from build123d import *

# Parameters (mm, degrees)
F0_W      = 50
F0_H      = 90
F1_DEPTH  = 50
F3_DEPTH  = 90.001
F4_R      = 8.198492098
F5_DEPTH  = 50.001
F6_R      = 10.8639610307
F8_DEPTH  = 50.001
F11_DEPTH = 90.001
F13_DEPTH = 90.0010001
F14_DEPTH = 90.0010001
F15_DEPTH = 27


with BuildPart() as f1:
    # F0 (on Top) → F1 (new body)
    with BuildSketch(Plane.XY):
        Rectangle(F0_W, F0_H)
    extrude(amount=F1_DEPTH)

    # F2 (on face) → F3 (cut, through all)
    with BuildSketch(Plane.XZ.offset(45)):
        Polygon((0, 25), (-25, 0), (25, 0), align=None)
    extrude(amount=-F3_DEPTH, mode=Mode.SUBTRACT)

    # F4 (on face) → F5 (cut, through all)
    with BuildSketch(Plane(origin=(-25, 0, 0), x_dir=(0, -1, 0), z_dir=(-1, 0, 0))):
        with Locations((-33.659145236, 38.9719307423)):
            Circle(F4_R)
    extrude(amount=-F5_DEPTH, mode=Mode.SUBTRACT)

    # F6
    f6_edges = [f1.edges().sort_by_distance(p)[0] for p in [
        (0, 45, 50),
    ]]
    fillet(f6_edges, radius=F6_R)

    # F7 (on face) → F8 (cut, through all)
    with BuildSketch(Plane.YZ.offset(25)):
        Polygon((28.1980223954, 0), (45, 0), (45, 29.2644444853), align=None)
    extrude(amount=-F8_DEPTH, mode=Mode.SUBTRACT)

    # F10 (on face) → F11 (cut, through all)
    with BuildSketch(Plane.XZ.offset(45)):
        with BuildLine():
            add(Edge.make_bspline(
                [(0, 46.1721457541), (-10.2533935373, 46.1721457541), (-5.1266967687, 31.8932551891), (0, 17.614364624), (5.1266967687, 31.8932551891), (10.2533935373, 46.1721457541), (0, 46.1721457541)],
                knots=[0, 0, 0, 2.0943951024, 2.0943951024, 4.1887902048, 4.1887902048, 6.2831853072, 6.2831853072, 6.2831853072], degree=2, weights=[1, 0.5, 1, 0.5, 1, 0.5, 1]))
        make_face()
    extrude(amount=-F11_DEPTH, mode=Mode.SUBTRACT)

    # F12 (on face) → F13 (cut, through all)
    with BuildSketch(Plane.XZ.offset(45)):
        Polygon((25, 7.2744810022), (17.7255189978, 7.2744810022), (25, 0), align=None)
        Polygon((-17.7255189978, 7.2744810022), (-25, 7.2744810022), (-25, 0), align=None)
    extrude(amount=-F13_DEPTH, mode=Mode.SUBTRACT)

    # F9 (on face) → F14 (cut, through all)
    with BuildSketch(Plane.XZ.offset(45)):
        Polygon((25, 10.9673021361), (25, 46.2542101741), (10.0381237455, 25.9291783907), align=None)
        Polygon((-25, 46.2542101741), (-25, 10.9673021361), (-10.0381237455, 25.9291783907), align=None)
    extrude(amount=-F14_DEPTH, mode=Mode.SUBTRACT)

    # F15 (cut): a face of the model
    f15_faces = [f1.faces().sort_by_distance(p)[0] for p in [
        (21.3627594989, -45, 7.9321640574),
    ]]
    extrude(f15_faces, amount=-F15_DEPTH, mode=Mode.SUBTRACT)


solid = f1.part
Build history of the part. All positions in model axes, mm. A direction names the side the tool comes from. Round coordinates to 2 decimals unless told otherwise and drop trailing zeros. Write each loop counter-clockwise with the first axis right and the second up, starting at its lowest first coordinate (ties: lowest second). Pieces come first, ordered by that corner, then holes. Notation, with made-up numbers: M 17.25,5.5 L 75.25,5.5 A18 ccw 75.25,29.5 Z; hole C 3.25,3 d7. An arc over 180 degrees is marked long. Answer as a JSON object with one key per item and string values. Group by question number.
(1) Cut at B-B (z = 16). Give the cut face in (x, y), and give its area (3 significant figures).
(2) Cut at D-D (x = -22). Give the cut face in (y, z), and give its area (3 significant figures).
(3) Drill centre lines: L1, parallel to Z at x = -11, y = 27; L2, parallel to Z at x = 12.5, y = 27; L3, parallel to X at y = 41, z = 33.5. Where is each one in solid material? Low to high.
(4) Flat gauge pins, fed straight in: pin 1 (4 mm diameter, centred on y = -8, z = 30, fed in from +X); pin 2 (10 mm diameter, centred on y = 33.66, z = 38.97, fed in from -X); pin 3 (4 mm diameter, centred on x = 15, y = -7, fed in from -Z); pin 4 (1.5 mm diameter, centred on x = -7.5, y = 8, fed in from -Z). Where does each tip first touch, or does it go through?
(5) Which spindle directions (+Z, -Z, +X, -X, +Y, -Y) get a long thin tool onto all of the face, cutting with end or side? Do faces 1 (the flat face through (-17.414, 6.059, 35.949)), 2 (the flat face through (17.414, 12.115, 18.553)), 3 (the flat face through (9, 12, 16)). Say none if no direction does.
(6) Cut at A-A (x = 16). Give the cut face in (y, z), and give its area (3 significant figures).
(7) Cut at C-C (x = 7.5). Give the cut face in (y, z), and give its area (3 significant figures).
(8) Mould opens along Z. For faces 4 (the cylindrical face through (-0.35, 34.73, 47.1)), 5 (the flat face through (0, 8, 50)), 6 (the flat face through (-10, 45, 34)) say: pulls with the +Z half, pulls with the -Z half, needs draft (parallel to the pull), parting line crosses it, or undercut.
Responses:
{
 "1": {"outline": "M -19.97,-18 L -9,-18 L -9,37.38 L -19.97,37.38 Z; M 9,-18 L 19.97,-18 L 19.97,37.38 L 9,37.38 Z", "area": "1,210 mm2"},
 "2": {"outline": "M -18,7.27 L 32.37,7.27 L 36.22,13.97 L -18,13.97 Z; M -18,42.18 L 26.11,42.18 A8.2 cw 41.2,42.18 L 44.57,42.18 A10.86 ccw 34.14,50 L -18,50 Z", "area": "763 mm2"},
 "3": {"L1": "z = 14 to 24.97, 27.24 to 34.19, 43.75 to 50", "L2": "z = 12.5 to 23.47, 29.27 to 34.19, 43.75 to 50", "L3": "x = -15.61 to -5.59, 5.59 to 15.61"},
 "4": {"pin 1": "stops at x = 14.51", "pin 2": "passes through", "pin 3": "stops at z = 8", "pin 4": "stops at z = 16.75"},
 "5": {"face 1": "-X, +Y, -Y", "face 2": "+X, +Y, -Y", "face 3": "-Z, +Y, -Y"},
 "6": {"outline": "M -18,9 L 33.37,9 L 39.66,19.97 L -18,19.97 Z; M -18,34.03 L 27.12,34.03 A8.2 cw long 40.2,34.03 L 45,34.03 L 45,39.14 A10.86 ccw 34.14,50 L -18,50 Z", "area": "1,400 mm2"},
 "7": {"outline": "M -18,17.5 L 38.25,17.5 L 45,29.26 L 45,39.14 A10.86 ccw 34.14,50 L -18,50 Z; hole C 33.66,38.97 d16.4", "area": "1,770 mm2"},
 "8": {"face 4": "undercut", "face 5": "pulls with the +Z half", "face 6": "needs draft"}
}
